Autodesk Inventor part; units mm, degrees
ref_plane "YZ Plane" through (0, 0, 0) normal (1, 0, 0) x (0, 1, 0)
ref_plane "XZ Plane" through (0, 0, 0) normal (0, 1, 0) x (-1, 0, 0)
ref_plane "XY Plane" through (0, 0, 0) normal (0, 0, 1) x (1, 0, 0)
sketch "Sketch1" plane through (0, 0, 0) normal (0, 0, 1) x (1, 0, 0)
  line L0 (0, 0) -> (36, 0)
  line L1 (36, 0) -> (36, 12)
  line L2 (36, 12) -> (24, 12)
  line L3 (24, 12) -> (24, 22)
  line L4 (24, 22) -> (12, 22)
  line L5 (12, 22) -> (12, 12)
  line L6 (12, 12) -> (0, 12)
  line L7 (0, 12) -> (0, 0)
  dimension "d0" = 36
  dimension "d1" = 12
  dimension "d2" = 12
  dimension "d3" = 10
  dimension "d4" = 12
extrude "Extrusion1" add sketch "Sketch1" along normal blind 108
sketch "Sketch2" plane through (0, 0, 0) normal (0, -1, 0) x (1, 0, 0)
  circle A0 centre (18, 4.5) radius 1.725
  line L0 (0, 0) -> (36, 0)
  line L1 (36, 0) -> (36, 108)
  circle A1 centre (18, 103.5) radius 1.725
  line L2 (0, 108) -> (36, 108)
  dimension "d7" = 3.45
  dimension "d8" = 4.5
  dimension "d9" = 18
  dimension "d10" = 3.45
  dimension "d11" = 18
  dimension "d12" = 4.5
extrude "Extrusion2" cut sketch "Sketch2" against normal blind 20
sketch "Sketch3" plane through (12, 22, 0) normal (0, 1, 0) x (1, 0, 0)
  circle A0 centre (6, -4.5) radius 1.725
  circle A1 centre (6, -4.5) radius 3
  circle A2 centre (6, -103.5) radius 1.725
  circle A3 centre (6, -103.5) radius 3
  point P0 (-12, 0)
  dimension "d15" = 6
  dimension "d16" = 6
extrude "Extrusion3" cut sketch "Sketch3" against normal blind 2 contours A0 | A1 | A2 | A3
sketch "Sketch4" plane through (36, 0, 0) normal (1, 0, 0) x (0, 0, -1)
  line L0 (-108, 0) -> (-107.85, 0)
  line L1 (0, 0) -> (-108, 0)
  line L2 (-107.85, 0) -> (-107.85, 12)
  line L3 (0, 12) -> (-108, 12)
  line L4 (-108, 0) -> (-108, 12)
  line L5 (-108, 12) -> (-108, 0)
  line L6 (-108, 22) -> (-107.85, 22)
  line L7 (-107.85, 12) -> (-108, 12)
  line L8 (0, 0) -> (-0.15, 0)
  line L9 (-0.15, 0) -> (-0.15, 12)
  line L10 (-0.15, 12) -> (0, 12)
  line L11 (0, 12) -> (0, 0)
  line L12 (0, 22) -> (-0.15, 22)
  line L13 (-0.15, 12) -> (0, 12)
  dimension "d19" = 0.15
  dimension "d20" = 12
  dimension "d21" = 0.15
  dimension "d22" = 0.15
extrude "Extrusion4" cut sketch "Sketch4" against normal through all contours L4 L3 L2 L0 | L9 L3 L11 L1
sketch "Sketch5" plane through (24, 22, 108) normal (1, 0, 0) x (0, 0, -1)
  line L0 (108, -10) -> (108, 0)
  line L1 (108, 0) -> (0, 0)
  line L2 (108, -10) -> (107.85, -10)
  line L3 (107.85, -10) -> (107.85, 0)
  line L4 (107.85, 0) -> (108, 0)
  line L5 (108, 0) -> (108, -10)
  line L6 (0.15, -10) -> (0, -10)
  line L7 (0, -10) -> (0, 0)
  line L8 (0.15, -10) -> (0, -10)
  line L9 (0, -10) -> (0, 0)
  line L10 (0, 0) -> (0.15, 0)
  line L11 (0.15, 0) -> (0.15, -10)
  point P0 (108, -22)
  dimension "d25" = 0.15
extrude "Extrusion5" cut sketch "Sketch5" against normal through all
sketch "Sketch6" plane through (12, 22, 0.15) normal (0, 1, 0) x (1, 0, 0)
  line L0 (0, 0) -> (0, -107.7)
  line L1 (12, 0) -> (12, -107.7)
  line L2 (0, -98.85) -> (12, -98.85)
  line L3 (12, -98.85) -> (12, -8.85)
  line L4 (12, -8.85) -> (0, -8.85)
  line L5 (0, -8.85) -> (0, -98.85)
  point P0 (-12, 0.15)
  dimension "d28" = 8.85
  dimension "d29" = 8.85
sketch "Sketch7" plane through (0, 0, 107.85) normal (0, -1, 0) x (1, 0, 0)
  line L0 (0, -107.7) -> (36, -107.7)
  line L1 (11.85, -107.7) -> (24.15, -107.7)
  line L2 (24.15, -107.7) -> (24.15, -98.55)
  line L3 (24.15, -98.55) -> (11.85, -98.55)
  line L4 (11.85, -98.55) -> (11.85, -107.7)
  line L5 (0, 0) -> (12, 0)
  line L6 (11.85, 0) -> (24.15, 0)
  line L7 (24.15, 0) -> (24.15, -9.15)
  line L8 (24.15, -9.15) -> (11.85, -9.15)
  line L9 (11.85, -9.15) -> (11.85, 0)
  line L10 (36, -107.7) -> (36, 0)
  point P0 (0, -107.85)
  dimension "d30" = 11.85
  dimension "d31" = 11.85
  dimension "d32" = 9.15
  dimension "d33" = 11.85
  dimension "d34" = 11.85
  dimension "d35" = 9.15
extrude "Extrusion6" cut sketch "Sketch7" against normal blind 6
sketch "Sketch8" plane through (36, 0, 0.15) normal (0, -1, 0) x (1, 0, 0)
  line L0 (-21, 95.7) -> (-15, 95.7)
  line L1 (-15, 95.7) -> (-15, 12)
  line L2 (-15, 12) -> (-21, 12)
  line L3 (-21, 12) -> (-21, 95.7)
  line L4 (-11.85, 0) -> (-24.15, 0)
  line L5 (0, 107.7) -> (-11.85, 107.7)
  line L6 (-24, 0) -> (-24, 107.7)
  line L7 (-12, 0) -> (-12, 107.7)
  point P0 (-36, -0.15)
  dimension "d38" = 12
  dimension "d39" = 12
  dimension "d40" = 3
  dimension "d41" = 3
extrude "Extrusion7" cut sketch "Sketch8" against normal through all
sketch "Sketch9" plane through (24, 12, 107.85) normal (0, 1, 0) x (1, 0, 0)
  line L0 (9, 3) -> (0, 3)
  line L1 (0, 3) -> (0, 104.7)
  line L2 (0, 104.7) -> (9, 104.7)
  line L3 (9, 104.7) -> (9, 3)
  line L4 (-12, 3) -> (-21, 3)
  line L5 (-21, 3) -> (-21, 104.7)
  line L6 (-21, 104.7) -> (-12, 104.7)
  line L7 (-12, 104.7) -> (-12, 3)
  line L8 (12, 0) -> (0.15, 0)
  line L9 (12, 107.7) -> (0, 107.7)
  line L10 (12, 107.7) -> (12, 0)
  line L11 (-24, 107.7) -> (-24, 0)
  line L12 (-12, 107.7) -> (-24, 107.7)
  line L13 (-24, 0) -> (-12, 0)
  line L14 (-12, 107.7) -> (-12, 0)
  line L15 (0, 107.7) -> (0, 0)
  point P0 (-24, 107.85)
  dimension "d44" = 3
  dimension "d45" = 3
  dimension "d46" = 3
  dimension "d47" = 3
  dimension "d48" = 3
  dimension "d49" = 3
  dimension "d50" = 0
  dimension "d51" = 0
extrude "Extrusion8" cut sketch "Sketch9" against normal through all contours L0 L1 L2 L3 | L4 L5 L6 L7
sketch "Sketch10" plane through (12, 0, 98.7) normal (0, -1, 0) x (1, 0, 0)
  line L0 (3, -86.55) -> (3, -2.85)
  line L1 (9, -2.85) -> (9, -86.55)
  line L2 (3, -2.85) -> (9, -2.85)
  line L3 (9, -2.85) -> (9, -86.55)
  line L4 (9, -86.55) -> (3, -86.55)
  line L5 (3, -86.55) -> (3, -2.85)
  line L6 (0, 0) -> (0, -89.4)
  line L7 (12, -98.55) -> (12, 9.15)
  line L8 (0, 0) -> (12, 0)
  line L9 (12, 0) -> (12, -89.4)
  line L10 (12, -89.4) -> (0, -89.4)
  line L11 (0, -89.4) -> (0, 0)
  line L12 (12, -89.4) -> (0, -89.4)
  line L13 (0, -89.4) -> (0, 0)
  line L14 (0, 0) -> (12, 0)
  line L15 (12, 0) -> (12, -89.4)
  point P0 (-12, -98.7)
sketch "Sketch11" plane through (36, 0, 107.85) normal (0, 0, 1) x (1, 0, 0)
  line L0 (-36, 0) -> (-36, 12)
  line L1 (-24.15, 0) -> (-33, 0)
  line L2 (-36, 12) -> (-24.15, 12)
  line L3 (-24.15, 12) -> (-24.15, 0)
  line L4 (-24.15, 0) -> (-36, 0)
  line L5 (-36, 0) -> (-36, 12)
extrude "Extrusion9" cut sketch "Sketch11" against normal through all
sketch "Sketch12" plane through (36, 0, 0.15) normal (0, 0, -1) x (-1, 0, 0)
  line L0 (24, 12) -> (24, 22)
  line L1 (24.15, 6) -> (24.15, 12)
  line L2 (24, 12) -> (24.15, 12)
  line L3 (24.15, 12) -> (24.15, 6)
  line L4 (24.15, 6) -> (24, 6)
  line L5 (24, 6) -> (24, 12)
  point P0 (36, 0)
extrude "Extrusion10" cut sketch "Sketch12" against normal through all
properties part number "cutcenterbeam"
Design review of the part built by this model. Coordinates are the model's own, in mm. A direction names the side the tool comes from. Give positions to 0.01 mm unless a question says otherwise; leave off trailing zeros. Loops run counter-clockwise (first coordinate to the right, second up) from the corner with the lowest first, then second, coordinate; pieces in that order, holes last. Notation, with made-up numbers: M 52,-25 L 95,-25 A19 cw 95,-5 Z; hole C 87,53 d3. An arc over 180 degrees is marked long. Write item = value, one per line.
Q1. We need section C-C (z = 4.5). Give the boundary of the cut face in (x, y) (3 decimals), plus the area to 3 significant figures.
Output values:
outline = M 12,6 L 16.275,6 L 16.275,20 L 15,20 L 15,22 L 12,22 Z; M 19.725,6 L 24,6 L 24,22 L 21,22 L 21,20 L 19.725,20 Z; M 33,0 L 36,0 L 36,12 L 33,12 Z
area = 168 mm^2
Q2. For faces 4 (the flat face through (20, 20, 103)), 5 (the flat face through (18, 11, 95.85)), 6 (the flat face through (24.15, 3, 106)), list the 3-axis set-ups (+Z, -Z, +X, -X, +Y, -Y) from which the entire face can be reached by the end or side of a thin tool; tool diameter is ignored.
Output values:
face_4 = +Y
face_5 = +Y, -Y
face_6 = +Z, -Z, -X, -Y
Q3. To check wall thickness, follow line 1 (Z direction, x = 18, y = 11.75) (3 decimals); line 2 (X direction, y = 11, z = 103.5) (3 decimals); line 3 (Z direction, x = 18, y = 21). State the ranges of each line that lie inside material, in increasing order. Write a range as [from, to].
Output values:
line_1 = [0.15, 2.775], [6.225, 12.15], [95.85, 101.775], [105.225, 107.85]
line_2 = [12, 16.275], [19.725, 24], [33, 36]
line_3 = [0.15, 1.5], [7.5, 12.15], [95.85, 100.5], [106.5, 107.85]
Q4. We need section B-B (x = 29.5). Give the boundary of the cut face in (y, z).
Output values:
outline = M 0,0.15 L 12,0.15 L 12,3.15 L 0,3.15 Z; M 0,104.85 L 12,104.85 L 12,107.85 L 0,107.85 Z
Q5. Draft analysis for pull direction X (two halves, no side actions). For faces 1 (the flat face through (24, 11, 107.85)), 2 (the flat face through (24.15, 3, 2)), 3 (the flat face through (15, 11, 53)), state which applies: +X half, -X half, draft (parallel to the pull), parting line (faces both ways), or undercut.
Output values:
face_1 = draft
face_2 = -X half
face_3 = undercut
Q6. We need section D-D (y = 15.25). Give the boundary of the cut face in (x, z) (3 decimals), plus the area to 3 significant figures.
Output values:
outline = M 12,0.15 L 24,0.15 L 24,107.85 L 12,107.85 Z; hole M 15,12.15 L 21,12.15 L 21,95.85 L 15,95.85 Z; hole C 18,4.5 d3.45; hole C 18,103.5 d3.45
area = 772 mm^2
Q7. We need section A-A (y = 3). Give the boundary of the cut face in (x, z), plus the area to 3 significant figures.
Output values:
outline = M 12,9.3 L 24,9.3 L 24,98.7 L 12,98.7 Z; M 24.15,0.15 L 36,0.15 L 36,107.85 L 24.15,107.85 L 24.15,104.85 L 33,104.85 L 33,3.15 L 24.15,3.15 Z; hole M 15,12.15 L 21,12.15 L 21,95.85 L 15,95.85 Z
area = 947 mm^2
Q8. Insertion check: pin 1 (5 mm diameter, centred on x = 16.5, y = 2, fed in from -Z); pin 2 (3 mm diameter, centred on x = 18, z = 4.5, fed in from +Y); pin 3 (0.9 mm diameter, centred on y = 4.5, z = 106.5, fed in from -X); pin 4 (5 mm diameter, centred on y = 19.5, z = 75, fed in from +X). Each pin has a flat end and moves straight along its axis. Give the tip position at first contact, or say it passes through.
Output values:
pin_1 = 9.3
pin_2 = through
pin_3 = 24.15
pin_4 = 24
